from build123d import *

# Parameters (mm, degrees)
SKETCH1_W                              = 165.1
SKETCH1_H                              = 165.1
BOSS_EXTRUDE1_DEPTH                    = 38.1
BOSS_EXTRUDE1_DEPTH_BACK               = 2
SKETCH2_W                              = 95.25
SKETCH2_H                              = 95.25
BOSS_EXTRUDE2_DEPTH                    = 38.1
BOSS_EXTRUDE3_START                    = -95.25
BOSS_EXTRUDE3_DEPTH                    = 95.25
SKETCH7_R                              = 12.7
CUT_EXTRUDE1_DEPTH                     = 131.175
SKETCH8_W                              = 38.1
SKETCH8_H                              = 1000
CUT_EXTRUDE2_DEPTH                     = 131.175
FILLET1_R                              = 3.175
SKETCH9_R                              = 26
CUT_EXTRUDE3_DEPTH                     = 36.83
SKETCH10_R                             = 76.2
SKETCH10_R_2                           = 69.85
CUT_EXTRUDE4_DEPTH                     = 8
F_1_2_14_NPSM_TAPPED_HOLE2_D           = 18.9738
F_1_2_14_NPSM_TAPPED_HOLE2_DEPTH       = 63.5
F_1_2_14_NPSM_TAPPED_HOLE2_CSINK_D     = 22.1742
F_1_2_14_NPSM_TAPPED_HOLE2_CSINK_ANGLE = 90
F_1_2_14_NPSM_TAPPED_HOLE2_TIP         = 5.700304607
SKETCH16_R                             = 6.35
CUT_EXTRUDE5_DEPTH                     = 25
SKETCH17_R                             = 6.35
CUT_EXTRUDE6_DEPTH                     = 126.825


with BuildPart() as part:
    # Sketch1 → Boss-Extrude1 (new body, two sides)
    with BuildSketch(Plane(origin=(0, 0, 0), x_dir=(1, 0, 0), z_dir=(0, 1, 0))) as boss_extrude1_sk:
        Rectangle(SKETCH1_W, SKETCH1_H)
    extrude(amount=BOSS_EXTRUDE1_DEPTH)
    extrude(boss_extrude1_sk.sketch, amount=-BOSS_EXTRUDE1_DEPTH_BACK)

    # Sketch2 → Boss-Extrude2 (add)
    with BuildSketch(Plane(origin=(0, 38.1, 0), x_dir=(1, 0, 0), z_dir=(0, 1, 0))):
        Rectangle(SKETCH2_W, SKETCH2_H)
    extrude(amount=BOSS_EXTRUDE2_DEPTH)

    # Sketch3 → Boss-Extrude3 (add)
    with BuildSketch(Plane(origin=(0, 0, -47.625), x_dir=(-1, 0, 0), z_dir=(0, 0, -1)).offset(BOSS_EXTRUDE3_START)):
        with BuildLine():
            Line((47.625, 76.2), (-47.625, 76.2))
            ThreePointArc((-47.625, 76.2), (0, 123.825), (47.625, 76.2))
        make_face()
    extrude(amount=BOSS_EXTRUDE3_DEPTH)

    # Sketch7 → Cut-Extrude1 (cut, through all)
    with BuildSketch(Plane(origin=(0, 0, -47.625), x_dir=(-1, 0, 0), z_dir=(0, 0, -1))):
        with Locations((0, 76.2)):
            Circle(SKETCH7_R)
    extrude(amount=-CUT_EXTRUDE1_DEPTH, mode=Mode.SUBTRACT)

    # Sketch8 → Cut-Extrude2 (cut, through all)
    with BuildSketch(Plane(origin=(47.625, 0, 0), x_dir=(0, 0, -1), z_dir=(1, 0, 0))):
        with Locations((0, 538.1)):
            Rectangle(SKETCH8_W, SKETCH8_H)
    extrude(amount=-CUT_EXTRUDE2_DEPTH, mode=Mode.SUBTRACT)

    # Fillet1
    fillet1_edges = [part.edges().sort_by_distance(p)[0] for p in [
        (82.55, 18.05, 82.55),
        (-82.55, 18.05, 82.55),
        (-82.55, 18.05, -82.55),
        (82.55, 18.05, -82.55),
    ]]
    fillet(fillet1_edges, radius=FILLET1_R)

    # Sketch9 → Cut-Extrude3 (cut)
    with BuildSketch(Plane.XZ.offset(2)):
        Circle(SKETCH9_R)
    extrude(amount=-CUT_EXTRUDE3_DEPTH, mode=Mode.SUBTRACT)

    # Sketch10 → Cut-Extrude4 (cut)
    with BuildSketch(Plane.XZ.offset(2)):
        Circle(SKETCH10_R)
        Circle(SKETCH10_R_2, mode=Mode.SUBTRACT)
    extrude(amount=-CUT_EXTRUDE4_DEPTH, mode=Mode.SUBTRACT)

    # 1/2-14 NPSM Tapped Hole2
    with Locations(Plane(origin=(82.55, 0, 0), x_dir=(0, 0, -1), z_dir=(1, 0, 0))):
        with Locations((0, 18.05)):
            CounterSinkHole(F_1_2_14_NPSM_TAPPED_HOLE2_D / 2, F_1_2_14_NPSM_TAPPED_HOLE2_CSINK_D / 2, depth=F_1_2_14_NPSM_TAPPED_HOLE2_DEPTH, counter_sink_angle=F_1_2_14_NPSM_TAPPED_HOLE2_CSINK_ANGLE)
            with Locations((0, 0, -(F_1_2_14_NPSM_TAPPED_HOLE2_DEPTH + F_1_2_14_NPSM_TAPPED_HOLE2_TIP / 2))):  # 118° drill point
                Cone(0, F_1_2_14_NPSM_TAPPED_HOLE2_D / 2, F_1_2_14_NPSM_TAPPED_HOLE2_TIP, mode=Mode.SUBTRACT)

    # Sketch16 → Cut-Extrude5 (cut)
    with BuildSketch(Plane.XZ.offset(2)):
        with Locations((50.55, 0)):
            Circle(SKETCH16_R)
    extrude(amount=-CUT_EXTRUDE5_DEPTH, mode=Mode.SUBTRACT)

    # Sketch17 → Cut-Extrude6 (cut, through all)
    with BuildSketch(Plane.XZ.offset(2)):
        with Locations((-61.963767235, 61.963767235)):
            Circle(SKETCH17_R)
        with Locations((61.963767235, 61.963767235)):
            Circle(SKETCH17_R)
        with Locations((61.963767235, -61.963767235)):
            Circle(SKETCH17_R)
        with Locations((-61.963767235, -61.963767235)):
            Circle(SKETCH17_R)
    extrude(amount=-CUT_EXTRUDE6_DEPTH, mode=Mode.SUBTRACT)


solid = part.part
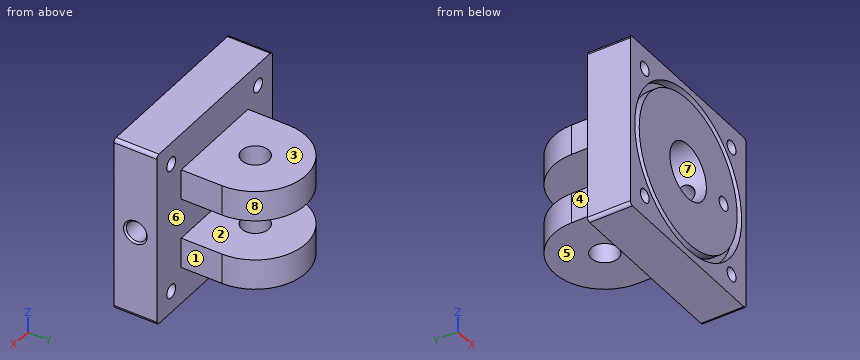
Work out the finished part from the listing and answer in its coordinate system (mm). Face numbers are marked on the shaded views. A direction names the side the tool comes from. Round coordinates to 2 decimals unless told otherwise and drop trailing zeros. Loops run counter-clockwise (first coordinate to the right, second up) from the corner with the lowest first, then second, coordinate; pieces in that order, holes last. Notation, with made-up numbers: M 39.25,83.5 L 66.25,83.5 A24 cw 66.25,117.5 Z; hole C 48,-32 d6. An arc over 180 degrees is marked long. One line per question, with ' | ' between items. Start each with the question number.
(1) A cutting plane is placed at A-A on y = 56. Write down the section's boundary in (x, z) (3 decimals).
(2) A tool of negligible diameter and unlimited length cuts with its end or side. For the marked faces 1, 2, 3, 4 and 5, from which of +Z, -Z, +X, -X, +Y, -Y can it reach the whole face along a straight path? Write none if from no direction.
(3) Flat-ended cylindrical pins translate along their axes: pin 1 Ø12 at (y, z) = (72, 56.5) entering from -X; pin 2 Ø12 at (x, z) = (65, 14) entering from +Y; pin 3 Ø5 at (x, z) = (-2, 6) entering from -Y; pin 4 Ø2 at (x, z) = (35.5, -61) entering from -Y. Find the tip coordinate at first contact, or state that the pin passes through.
(4) A cutting plane is placed at C-C on z = 0. Write down the section's boundary in (x, y), plus the area to 3 significant figures.
(5) A cutting plane is placed at D-D on y = 80.5. Write down the section's boundary in (x, z) (3 decimals), plus the area to 3 significant figures.
(6) Find the intervals of material crossed by line 1 (Z direction, x = 18, y = 89) (3 decimals); line 2 (Z direction, x = 66, y = 18); line 3 (Z direction, x = 50.5, y = 18.05), in increasing order.
(7) A cutting plane is placed at B-B on x = 0. Give the number of separate pieces and of enclosed holes in the cut face, plus the area to 3 significant figures.
(8) For a pull along X with two mould halves and no side action, classify the marked faces 6, 7 and 8 as released by +X, released by -X, zero draft, split by the parting line, or undercut.
Geometry check:
1) outline: M -47.625,-47.625 L 47.625,-47.625 L 47.625,-19.05 L -47.625,-19.05 Z; M -47.625,19.05 L 47.625,19.05 L 47.625,47.625 L -47.625,47.625 Z
2) face 1: +Z, -Z, +X, +Y | face 2: +X, -X, +Y | face 3: +Z, +X, -X, +Y | face 4: +Z, -Z, -X, +Y | face 5: -Z, +X, -X, +Y
3) pin 1: passes through | pin 2: stops at y = 38.1 | pin 3: stops at y = 34.83 | pin 4: stops at y = -2
4) outline: M -82.55,-2 L -76.2,-2 L -76.2,6 L -69.85,6 L -69.85,-2 L -26,-2 L -26,34.83 L 26,34.83 L 26,27.54 L 80.95,27.54 L 82.55,29.14 L 82.55,38.1 L -82.55,38.1 Z; M 26,-2 L 44.2,-2 L 44.2,8.56 L 26,8.56 Z; M 56.9,-2 L 69.85,-2 L 69.85,6 L 76.2,6 L 76.2,-2 L 82.55,-2 L 82.55,6.96 L 80.95,8.56 L 56.9,8.56 Z | area: 3,390 mm²
5) outline: M -47.43,-47.625 L -11.95,-47.625 L -11.95,-19.05 L -47.43,-19.05 Z; M -47.43,19.05 L -11.95,19.05 L -11.95,47.625 L -47.43,47.625 Z; M 11.95,-47.625 L 47.43,-47.625 L 47.43,-19.05 L 11.95,-19.05 Z; M 11.95,19.05 L 47.43,19.05 L 47.43,47.625 L 11.95,47.625 Z | area: 4,060 mm²
6) line 1: z = -47.625 to -19.05, 19.05 to 47.625 | line 2: z = -82.55 to -66.87, -57.06 to -9.49, 9.49 to 57.06, 66.87 to 82.55 | line 3: z = -82.55 to -9.49, 9.49 to 82.55
7) separate pieces: 3 | enclosed holes: 0 | area: 8,050 mm²
8) face 6: zero draft | face 7: undercut | face 8: split by the parting line
